Geometry: final body of the model. Coordinates: model frame, mm. Face numbers are marked on the shaded views. A direction names the side the tool comes from. Give positions to 0.01 mm unless a question says otherwise; leave off trailing zeros. Order: outer loops, then holes, each group sorted by start corner. A loop starts at its lowest first (then second) coordinate and runs counter-clockwise, first axis right, second up. Notation, with made-up numbers: (86, 83) -> (116, 83) arc R31 ccw to (116, 115) -> close; hole circle Ø11 at (-37, 43). An arc over 180 degrees is marked (long way). Answer in a Markdown table with one row per item. Add a question column.
Q1. Cut plane B-B on x = 27. Return the cut outline in (y, z), and give its area (3 significant figures).
Q2. Pull-direction query (X, two-part tool) for the marked faces 3, 4, 5 and 6; classes: +X half, -X half, draft (parallel to the pull), parting line (faces both ways), or undercut.
Q3. Set-up query: the marked faces 1 and 2. Return all of +Z, -Z, +X, -X, +Y, -Y with unobstructed straight access to the full face (end or side cutting, diameter ignored); none if empty.
Q4. Line query: line 1 along X through (y, z) = (-14, 15.5); line 2 along Z through (x, y) = (-47, -29.1); line 3 along Y through (x, z) = (-8.5, 31). Output: solid intervals per line, ascending. Write a range as from..to.
Q5. Contact query for flat-ended pins moving along their axis: P1, Ø1, axis at x = -29.5, z = 28, coming from the +Y side; P2, Ø4.5, axis at x = 54.5, z = 30.5, coming from the +Y side. Output: stop coordinate, or through.
Q6. Cut plane D-D on x = -21. Return the cut outline in (y, z).
Q7. Cut plane C-C on z = 40. Return the cut outline in (x, y).
Q8. Cut plane A-A on y = -8. Return the cut outline in (x, z), and give its area (3 significant figures).
from build123d import *

# Parameters (mm, degrees)
F0_R      = 8
F1_DEPTH  = 3
F2_W      = 3
F2_H      = 3
F2_W_2    = 134
F3_DEPTH  = 40
F4_W      = 3
F4_H      = 40
F5_DEPTH  = 134
F6_W      = 126
F6_H      = 3
F7_DEPTH  = 40
F8_R      = 1.5
F9_DEPTH  = 3
F10_R     = 8
F12_DEPTH = 40


with BuildPart() as f1:
    # F0 (on Top) → F1 (new body)
    with BuildSketch(Plane.XY):
        Polygon((-60, 33.034884), (-80, 33.034884), (-80, 18.034884), (-80, 0.034884), (-80, -2.965116), (-80, -17.965116), (-80, -29.965116), (60, -29.965116), (60, -24.965116), (60, -14.965116), (60, -9.965116), (60, -4.965116), (60, 0.034884), (60, 18.034884), (60, 33.034884), (40, 33.034884), (20, 33.034884), (0, 33.034884), (-20, 33.034884), (-40, 33.034884), align=None)
        with Locations((25, -0.468963)):
            Circle(F0_R, mode=Mode.SUBTRACT)
        with Locations((-45, 1.034884)):
            Circle(F0_R, mode=Mode.SUBTRACT)
    extrude(amount=F1_DEPTH)

    # F2 (on face) → F3 (join)
    with BuildSketch(Plane.XY.offset(3)):
        with Locations((-78.5, -28.465116)):
            Rectangle(F2_W, F2_H)
        with Locations((-10, -28.465116)):
            Rectangle(F2_W_2, F2_H)
        Polygon((-80, 30.034884), (-80, -26.965116), (-77, -26.965116), (-77, 33.034884), (-80, 33.034884), align=None)
        with Locations((58.5, -28.465116)):
            Rectangle(F2_W, F2_H)
        Polygon((57, 33.034884), (57, -26.965116), (60, -26.965116), (60, 30.034884), (60, 33.034884), align=None)
    extrude(amount=F3_DEPTH)

    # F4 (on face) → F5 (join)
    with BuildSketch(Plane.YZ.offset(-77)):
        with Locations((28.334884, 23)):
            Rectangle(F4_W, F4_H)
    extrude(amount=F5_DEPTH)

    # F6 (on face) → F7 (cut)
    with BuildSketch(Plane.XY.offset(43)):
        with Locations((-10, 28.334884)):
            Rectangle(F6_W, F6_H)
    extrude(amount=-F7_DEPTH, mode=Mode.SUBTRACT)

    # F8 (on face) → F9 (cut)
    with BuildSketch(Plane(origin=(0, -26.965116, 0), x_dir=(-1, 0, 0), z_dir=(0, 1, 0))):
        with Locations((47, 26.988985)):
            Circle(F8_R)
        with Locations((-27, 26.988985)):
            Circle(F8_R)
        with Locations((10, 26.988985)):
            Circle(F8_R)
    extrude(amount=-F9_DEPTH, mode=Mode.SUBTRACT)

    # F10 (on face) → F12 (cut)
    with BuildSketch(Plane.XY.offset(3)):
        Polygon((57, 29.834884), (57, 33.034884), (-77, 33.034884), (-77, 29.834884), (-73, 29.834884), (-73, 26.834884), (-77, 26.834884), (-77, -26.965116), (57, -26.965116), (57, 26.834884), (53, 26.834884), (53, 29.834884), align=None)
        with Locations((-45, 1.034884)):
            Circle(F10_R, mode=Mode.SUBTRACT)
        with Locations((25, -0.468963)):
            Circle(F10_R, mode=Mode.SUBTRACT)
    extrude(amount=-F12_DEPTH, mode=Mode.SUBTRACT)


solid = f1.part
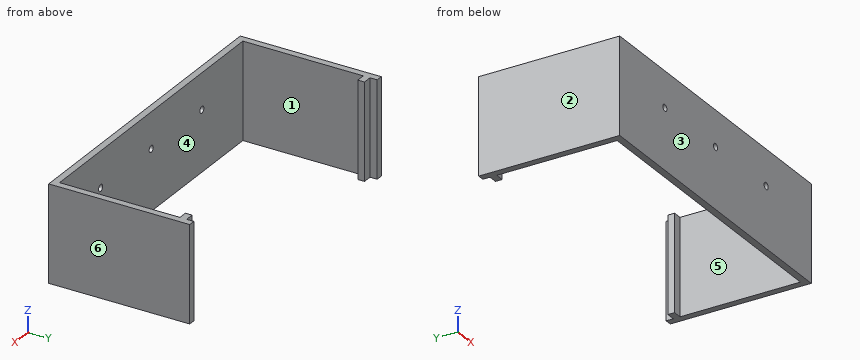
Completed:
| question | item | result |
|---|---|---|
| 1 | outline | (-29.97, 0) -> (-26.97, 0) -> (-26.97, 25.49) -> (-29.97, 25.49) -> close; (-29.97, 28.49) -> (-26.97, 28.49) -> (-26.97, 43) -> (-29.97, 43) -> close |
| 1 | area | 120 mm² |
| 2 | face 3 | draft |
| 2 | face 4 | undercut |
| 2 | face 5 | undercut |
| 2 | face 6 | +X half |
| 3 | face 1 | +Z, -Z |
| 3 | face 2 | +Z, -Z, -X, +Y, -Y |
| 4 | line 1 | x = -80..-77, 57..60 |
| 4 | line 2 | z = 0..25.49, 28.49..43 |
| 4 | line 3 | y = -29.97..-26.97 |
| 5 | P1 | stops at y = -26.97 |
| 5 | P2 | stops at y = 29.83 |
| 6 | outline | (-29.97, 0) -> (-26.97, 0) -> (-26.97, 43) -> (-29.97, 43) -> close |
| 7 | outline | (-80, -29.97) -> (60, -29.97) -> (60, 33.03) -> (57, 33.03) -> (57, 29.83) -> (53, 29.83) -> (53, 26.83) -> (57, 26.83) -> (57, -26.97) -> (-77, -26.97) -> (-77, 26.83) -> (-73, 26.83) -> (-73, 29.83) -> (-77, 29.83) -> (-77, 33.03) -> (-80, 33.03) -> close |
| 8 | outline | (-80, 0) -> (-77, 0) -> (-77, 43) -> (-80, 43) -> close; (57, 0) -> (60, 0) -> (60, 43) -> (57, 43) -> close |
| 8 | area | 258 mm² |
